The drawing under review shows one solid part. Ordinate dimensions are in mm from its lowest x, y, z. A direction names the side the tool comes from. Give positions to 0.01 mm unless a question says otherwise; leave off trailing zeros. Order: outer loops, then holes, each group sorted by start corner. A loop starts at its lowest first (then second) coordinate and runs counter-clockwise, first axis right, second up. Notation, with made-up numbers: (89, -9) - (141, -9) arc R19 cw to (141, 26) - close; hole circle Ø2 at (52, 6.25). An arc over 180 degrees is marked (long way). Use CSV: the item, a comma, the result in double quotes.
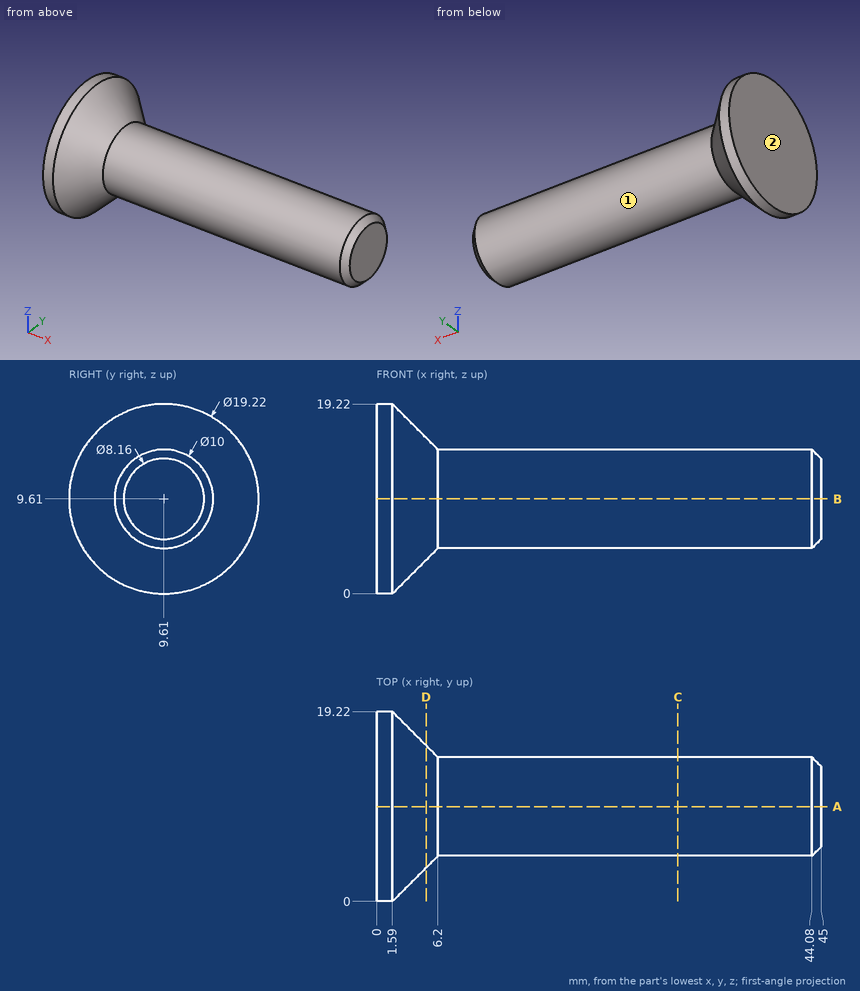
Item 1: Wall thickness on L1, parallel to X at y = 5, z = 9.5; L2, parallel to X at y = 6, z = 11.75 (1 decimal); L3, parallel to Y at x = 33, z = 9.25: over which ranges is each line inside the solid? List them lowest first.
Results list:
L1,"x = 0 to 44.47"
L2,"x = 0 to 44.9"
L3,"y = 4.62 to 14.6"
Item 2: Clearance check with flat-ended pins moving along their axes: pin 1 (1.5 mm diameter, centred on x = 28.5, y = 7, fed in from -Z); pin 2 (3 mm diameter, centred on x = 23.5, y = 10, fed in from -Z); pin 3 (2 mm diameter, centred on y = 12, z = 6, fed in from -X); pin 4 (4 mm diameter, centred on x = 8.5, z = 14.5, fed in from +Y). State where each tip first meets the part, or that it passes through.
Results list:
pin 1,"stops at z = 4.97"
pin 2,"stops at z = 4.61"
pin 3,"stops at x = 0"
pin 4,"stops at y = 13.69"
Item 3: Take a section at A-A, the plane y = 9.61. Give the boundary of the cut face in (x, z).
Results list:
outline,"(0, 0) - (1.59, 0) - (6.2, 4.61) - (44.08, 4.61) - (45, 5.53) - (45, 13.69) - (44.08, 14.61) - (6.2, 14.61) - (1.59, 19.22) - (0, 19.22) - close"
Item 4: Take a section at C-C, the plane x = 30.5. Give the boundary of the cut face in (y, z).
Results list:
outline,"circle Ø10 at (9.61, 9.61)"
Item 5: Take a section at D-D, the plane x = 5. Give the boundary of the cut face in (y, z).
Results list:
outline,"circle Ø12.4 at (9.61, 9.61)"
Item 6: Tool access review of the marked faces 1 and 2: name each direction out of +Z, -Z, +X, -X, +Y, -Y from which nothing blocks a thin tool from reaching the whole face with its end or side.
Results list:
face 1,"+X"
face 2,"+Z, -Z, -X, +Y, -Y"
